```python
from build123d import *

# Parameters (mm, degrees)
SKETCH2_R             = 19.05
EXTRUDE1_DEPTH        = 20.32
SKETCH4_W             = 35.2806
SKETCH4_H             = 35.2806
EXTRUDE2_DEPTH        = 21.59
SKETCH5_R             = 7.0866
EXTRUDE3_DEPTH        = 36.241069791
SKETCH7_R             = 7.62
EXTRUDE4_DEPTH        = 5.08
F_8_CLEARANCE_HOLE1_D = 4.3053


with BuildPart() as part:
    # Sketch2 → Extrude1 (new, symmetric)
    with BuildSketch(Plane.XY):
        Circle(SKETCH2_R)
    extrude(amount=EXTRUDE1_DEPTH, both=True)

    # Sketch4 → Extrude2 (cut)
    with BuildSketch(Plane(origin=(0, 19.05, 20.32), x_dir=(-1, 0, 0), z_dir=(0, 1, 0))):
        with Locations((0, -20.32)):
            Rectangle(SKETCH4_W, SKETCH4_H)
    extrude(amount=-EXTRUDE2_DEPTH, mode=Mode.SUBTRACT)

    # Sketch5 → Extrude3 (cut, through all)
    with BuildSketch(Plane(origin=(0, -2.54, 0), x_dir=(1, 0, 0), z_dir=(0, 1, 0))):
        with Locations(Location((0, 0, 0), (0, 0, 270))):
            Circle(SKETCH5_R)
    extrude(amount=-EXTRUDE3_DEPTH, mode=Mode.SUBTRACT)

    # Sketch7 → Extrude4 (add)
    with BuildSketch(Plane(origin=(0, 0, -20.32), x_dir=(-1, 0, 0), z_dir=(0, 0, -1))):
        with Locations(Location((0, 0, 0), (0, 0, 180))):
            Circle(SKETCH7_R)
    extrude4 = extrude(amount=EXTRUDE4_DEPTH)

    # Mirror1: Extrude4 across plane
    add(extrude4.mirror(Plane.XY))

    # #8 Clearance Hole1 (through all)
    with Locations(Plane(origin=(0, 0, -20.32), x_dir=(-1, 0, 0), z_dir=(0, 0, -1))):
        with Locations((-8.89, 10.16), (8.89, 10.16)):
            Hole(F_8_CLEARANCE_HOLE1_D / 2)


solid = part.part
```
Design review of the part built by this model. Coordinates are the model's own, in mm. A direction names the side the tool comes from. Round coordinates to 2 decimals unless told otherwise and drop trailing zeros. Order: outer loops, then holes, each group sorted by start corner. A loop starts at its lowest first (then second) coordinate and runs counter-clockwise, first axis right, second up. Notation, with made-up numbers: (45.25, -31) - (49.25, -31) arc R24 ccw to (49.25, -21) - close; hole circle Ø8 at (75.25, -24.5). An arc over 180 degrees is marked (long way). Return JSON: item names as keys, results as strings.
Q1. The part is to be moulded in two halves that separate along X. For faces 1 (the cylindrical face through (-0.992, -7.555, 22.824)), 2 (the flat face through (0, -8, -20.32)), 3 (the cylindrical face through (-9.17, 12.294, 18.999)), say which applies: pulls with the +X half, pulls with the -X half, needs draft (parallel to the pull), parting line crosses it, or undercut.
Computed values:
{"face 1": "parting line crosses it", "face 2": "needs draft", "face 3": "undercut"}
Q2. Consider section B-B on y = 3. Write out the cut boundary in (x, z).
Computed values:
{"outline": "(-18.81, -20.32) - (-7, -20.32) - (-7, -25.4) - (7, -25.4) - (7, -20.32) - (18.81, -20.32) - (18.81, 20.32) - (7, 20.32) - (7, 25.4) - (-7, 25.4) - (-7, 20.32) - (-18.81, 20.32) - close; hole (-17.64, -17.64) - (17.64, -17.64) - (17.64, 17.64) - (-17.64, 17.64) - close"}
Q3. Consider section A-A on z = 0. Write out the cut boundary in (x, y), plus the area to 3 significant figures.
Computed values:
{"outline": "(-17.64, -2.54) - (-17.64, 7.19) arc R19.05 ccw to (-7.09, -17.68) - (-7.09, -2.54) - close; (7.09, -17.68) arc R19.05 ccw to (17.64, 7.19) - (17.64, -2.54) - (7.09, -2.54) - close", "area": "266 mm2"}
Q4. For pin 1 Ø7 at (x, y) = (-8.89, 10.16) entering from +Z; pin 2 Ø6 at (y, z) = (5.5, 19.5) entering from -X; pin 3 Ø17.5 at (x, z) = (8, 7) entering from +Y, all flat-tipped, find the tip position at first contact; note any pin that passes through.
Computed values:
{"pin 1": "stops at z = 20.32", "pin 2": "stops at x = -18.89", "pin 3": "stops at y = -2.54"}
Q5. Consider section C-C on x = -9. Write out the cut boundary in (y, z).
Computed values:
{"outline": "(-16.79, -20.32) - (8.01, -20.32) - (8.01, -17.64) - (-2.54, -17.64) - (-2.54, 17.64) - (8.01, 17.64) - (8.01, 20.32) - (-16.79, 20.32) - close; (12.31, -20.32) - (16.79, -20.32) - (16.79, -17.64) - (12.31, -17.64) - close; (12.31, 17.64) - (16.79, 17.64) - (16.79, 20.32) - (12.31, 20.32) - close"}
Q6. Machinability: for faces 4 (the cylindrical face through (-0.992, -7.555, -22.824)), 5 (the flat face through (0, 0, -25.4)), 6 (the flat face through (0, 6, 17.64)), 7 (the cylindrical face through (8.61, 12.294, -18.961)), 8 (the flat face through (0, -8, 20.32)), which of the approach directions +Z, -Z, +X, -X, +Y, -Y give a long, thin tool a straight path to every point of the face, cutting with its end or side? Answer none if there is none.
Computed values:
{"face 4": "-Z", "face 5": "-Z, +X, -X, +Y, -Y", "face 6": "+Y", "face 7": "+Z, -Z", "face 8": "+Z"}
Q7. Consider section D-D on x = 5. Write out the cut boundary in (y, z), plus the area to 3 significant figures.
Computed values:
{"outline": "(-18.38, -20.32) - (-5.75, -20.32) - (-5.75, -25.4) - (5.75, -25.4) - (5.75, -20.32) - (18.38, -20.32) - (18.38, -17.64) - (-2.54, -17.64) - (-2.54, -5.02) - (-18.38, -5.02) - close; (-18.38, 5.02) - (-2.54, 5.02) - (-2.54, 17.64) - (18.38, 17.64) - (18.38, 20.32) - (5.75, 20.32) - (5.75, 25.4) - (-5.75, 25.4) - (-5.75, 20.32) - (-18.38, 20.32) - close", "area": "714 mm2"}
Q8. Wall thickness on L1, parallel to Z at x = 4, y = 14.5; L2, parallel to Y at x = -8.89, z = 19.6; L3, parallel to X at y = 10, z = -19: over which ranges is each line inside the solid? List them lowest first. Write a range as [from, to].
Computed values:
{"L1": "z = [-20.32, -17.64], [17.64, 20.32]", "L2": "y = [-16.85, 8.01], [12.31, 16.85]", "L3": "x = [-16.21, -11.04], [-6.74, 6.74], [11.04, 16.21]"}
